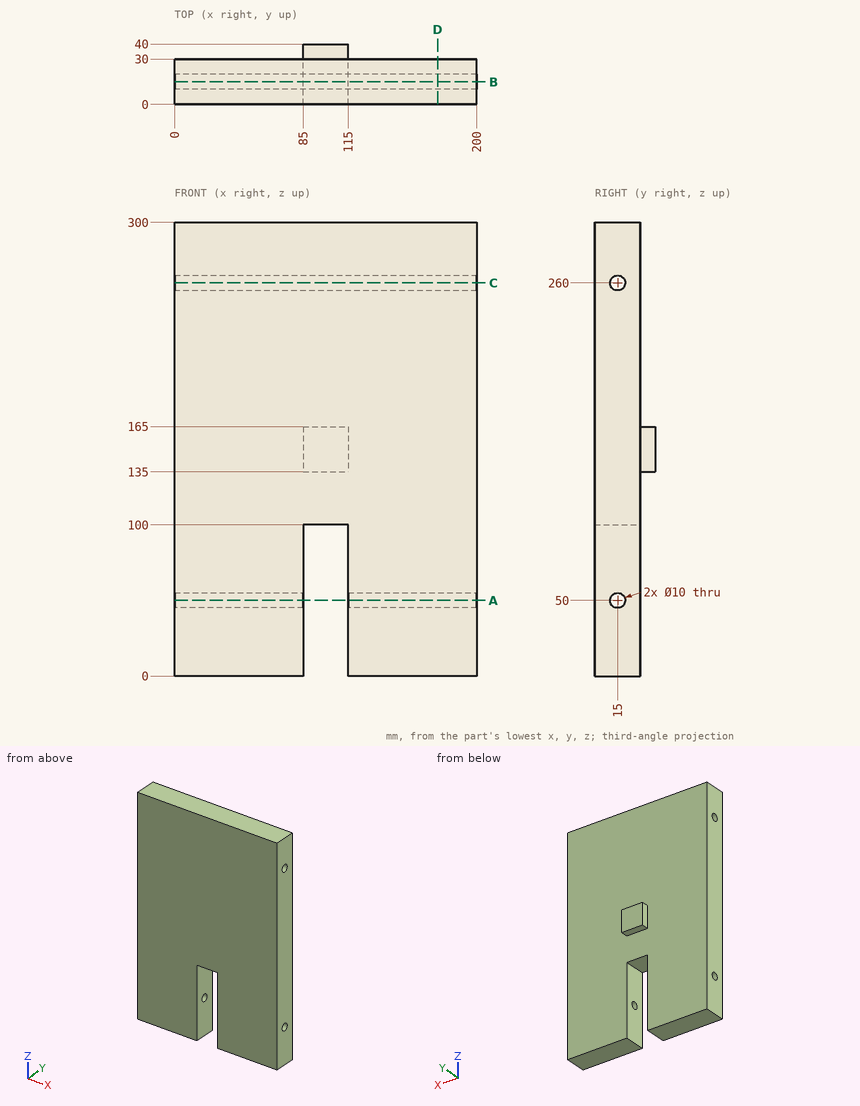
Design review of the part shown in the three views and the two pictorial views. Dimensions are in mm from the part's minimum x, y and z. Coordinates: 2 decimals unless noted, no trailing zeros. Write each loop counter-clockwise with the first axis right and the second up, starting at its lowest first coordinate (ties: lowest second). Pieces come first, ordered by that corner, then holes.
(1) Add section C-C on z = 260. Give the boundary of the cut face in (x, y), then the cut area to 3 significant figures.
(2) For pin 1 Ø9 at (x, y) = (107, 18) entering from -Z; pin 2 Ø5 at (y, z) = (33.5, 152) entering from +X; pin 3 Ø1.5 at (x, z) = (76, 79.5) entering from +Y, all flat-tipped, find the tip position at first contact; note any pin that passes through.
(3) Add section A-A on z = 50. Give the boundary of the cut face in (x, y), then the cut area to 3 significant figures.
(4) Wall thickness on probe 1 along X at (y, z) = (14.5, 87); probe 2 along Y at (x, z) = (27, 50); probe 3 along Z at (x, y) = (32.5, 18): over which ranges is each line inside the solid? List them lowest first.
(5) Add section B-B on y = 15. Give the boundary of the cut face in (x, z).
(6) Add section D-D on x = 174. Give the boundary of the cut face in (y, z).
Answer sheet:
1. outline: (0, 0) - (200, 0) - (200, 10) - (0, 10) - close; (0, 20) - (200, 20) - (200, 30) - (0, 30) - close
1. area: 4,000 mm2
2. pin 1: stops at z = 100
2. pin 2: stops at x = 115
2. pin 3: stops at y = 30
3. outline: (0, 0) - (85, 0) - (85, 10) - (0, 10) - close; (0, 20) - (85, 20) - (85, 30) - (0, 30) - close; (115, 0) - (200, 0) - (200, 10) - (115, 10) - close; (115, 20) - (200, 20) - (200, 30) - (115, 30) - close
3. area: 3,400 mm2
4. probe 1: x = 0 to 85, 115 to 200
4. probe 2: y = 0 to 10, 20 to 30
4. probe 3: z = 0 to 46, 54 to 256, 264 to 300
5. outline: (0, 0) - (85, 0) - (85, 45) - (0, 45) - close; (0, 55) - (85, 55) - (85, 100) - (115, 100) - (115, 55) - (200, 55) - (200, 255) - (0, 255) - close; (0, 265) - (200, 265) - (200, 300) - (0, 300) - close; (115, 0) - (200, 0) - (200, 45) - (115, 45) - close
6. outline: (0, 0) - (30, 0) - (30, 300) - (0, 300) - close; hole circle Ø10 at (15, 50); hole circle Ø10 at (15, 260)
